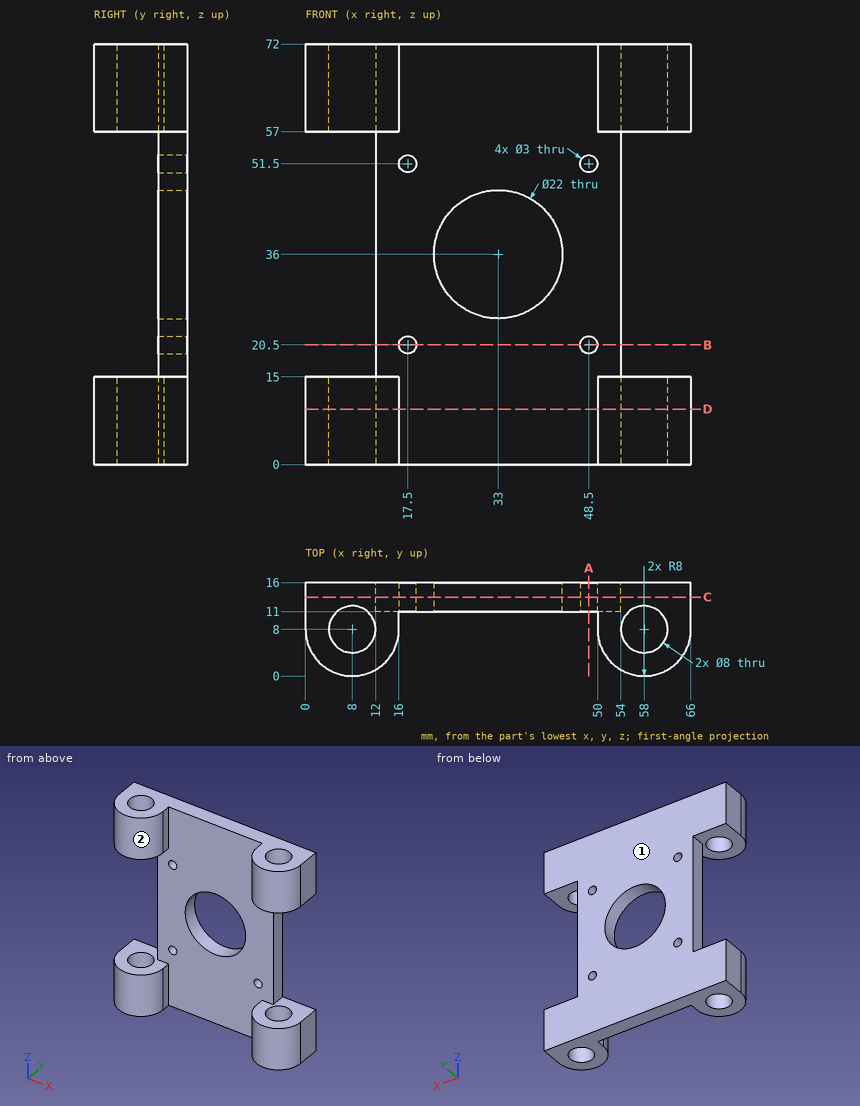
Geometry check sheet. Reference: drawing and pictorial views, mm from the part's lowest x, y, z. Coordinates: 2 decimals unless noted, no trailing zeros. Order: outer loops, then holes, each group sorted by start corner. A loop starts at its lowest first (then second) coordinate and runs counter-clockwise, first axis right, second up. Notation, with made-up numbers: (-1.75, 32) -> (5.25, 32) arc R26 cw to (5.25, 69) -> close; hole circle Ø4 at (66, -19.75). An arc over 180 degrees is marked (long way). Write item = value, one per line. Start each with the question number.
1) Cross-section at A-A (x = 48.5). Enter the section's corners in (y, z).
2) Material ranges on L1, parallel to X at y = 13.05, z = 51.5; L2, parallel to Z at x = 17.5, y = 15; L3, parallel to Y at x = 58, z = 8, recorded low to high.
3) Go/stop test with flat-tipped pins: P1, Ø17.5, axis at x = 33, z = 36, coming from the -Y side; P2, Ø3, axis at x = 38.5, z = 57, coming from the -Y side; P3, Ø5.5, axis at y = 12.5, z = 29.5, coming from the -X side; P4, Ø5.5, axis at y = 12.5, z = 32.5, coming from the +X side. Record where each tip stops, or that it passes through.
4) Mould release check, pull along X, two halves, no side actions. Record for the marked faces 1 and 2: +X half, -X half, draft (parallel to the pull), parting line (faces both ways), or undercut.
5) Cross-section at D-D (z = 9.5). Enter the section's corners in (x, y), then the cut area to 3 significant figures.
6) Cross-section at B-B (z = 20.5). Enter the section's corners in (x, y), then the cut area to 3 significant figures.
7) Cross-section at C-C (y = 13.5). Enter the section's corners in (x, z).
Ans:
q1.outline = (11, 0) -> (16, 0) -> (16, 19) -> (11, 19) -> close; (11, 22) -> (16, 22) -> (16, 50) -> (11, 50) -> close; (11, 53) -> (16, 53) -> (16, 72) -> (11, 72) -> close
q2.L1 = 12 to 16, 19 to 47, 50 to 54
q2.L2 = 0 to 19, 22 to 50, 53 to 72
q2.L3 = 0 to 4, 12 to 16
q3.P1 = through
q3.P2 = 11
q3.P3 = 12
q3.P4 = 54
q4.face_1 = draft
q4.face_2 = undercut
q5.outline = (0, 8) arc R8 ccw to (16, 8) -> (16, 11) -> (50, 11) -> (50, 8) arc R8 ccw to (66, 8) -> (66, 16) -> (0, 16) -> close; hole circle Ø8 at (8, 8); hole circle Ø8 at (58, 8)
q5.area = 527 mm²
q6.outline = (12, 11) -> (16, 11) -> (16, 16) -> (12, 16) -> close; (19, 11) -> (47, 11) -> (47, 16) -> (19, 16) -> close; (50, 11) -> (54, 11) -> (54, 16) -> (50, 16) -> close
q6.area = 180 mm²
q7.outline = (0, 0) -> (66, 0) -> (66, 15) -> (54, 15) -> (54, 57) -> (66, 57) -> (66, 72) -> (0, 72) -> (0, 57) -> (12, 57) -> (12, 15) -> (0, 15) -> close; hole circle Ø3 at (17.5, 20.5); hole circle Ø3 at (17.5, 51.5); hole circle Ø22 at (33, 36); hole circle Ø3 at (48.5, 20.5); hole circle Ø3 at (48.5, 51.5)
